Read the model definition and answer for the solid it produces. Units are mm, in the model's axes. A direction names the side the tool comes from. Coordinates: 2 decimals unless noted, no trailing zeros. Order: outer loops, then holes, each group sorted by start corner. A loop starts at its lowest first (then second) coordinate and runs counter-clockwise, first axis right, second up. Notation, with made-up numbers: (-24.5, 31) -> (30.5, 31) arc R26 cw to (30.5, 56) -> close; hole circle Ø4 at (50, -8). An arc over 180 degrees is marked (long way). Answer in a Markdown table with one row per item.
Autodesk Inventor part; units mm, degrees
ref_plane "YZ Plane" through (0, 0, 0) normal (1, 0, 0) x (0, 1, 0)
ref_plane "XZ Plane" through (0, 0, 0) normal (0, 1, 0) x (-1, 0, 0)
ref_plane "XY Plane" through (0, 0, 0) normal (0, 0, 1) x (1, 0, 0)
sketch "Sketch1" plane through (0, 0, 0) normal (0, 0, 1) x (1, 0, 0)
  line L0 (-50, 0) -> (50, 0)
  line L1 (0, 0) -> (0, 34.9563) construction
  line L2 (-50, 0) -> (-50, 10)
  line L3 (-50, 10) -> (50, 10)
  line L4 (50, 10) -> (50, 0)
  dimension "d0" = 100
  dimension "d1" = 10
revolve "Revolution1" add sketch "Sketch1" angle 360 about axis through (-50, 0, 0) along (1, 0, 0)
sketch "Sketch2" plane through (0, 0, 0) normal (0, 1, 0) x (-1, 0, 0)
  line L0 (-50, 10) -> (-50, -10)
  circle A0 centre (-50, 0) radius 17.5
  circle A1 centre (-50, 0) radius 10
  point P0 (0, 0)
  dimension "d3" = 35
  dimension "d4" = 20
extrude "Extrusion1" add sketch "Sketch2" along normal blind 20
extrude "Extrusion2" cut sketch "Sketch2" against normal blind 20 contours A1 L0 | A0 picked at (-47.9217, -2.6061)
extrude "Extrusion3" cut sketch "Sketch2" along normal blind 20 contours A1 L0 picked at (-47.9217, -2.6061)
sketch "Sketch4" plane through (0, 0, 0) normal (0, 1, 0) x (-1, 0, 0)
  line L0 (50, 10) -> (50, -10)
  circle A0 centre (50, 0) radius 17.5
  circle A1 centre (50, 0) radius 10
  point P0 (0, 0)
  dimension "d17" = 35
  dimension "d18" = 20
extrude "Extrusion6" add sketch "Sketch4" against normal blind 20
extrude "Extrusion7" cut sketch "Sketch4" along normal blind 20 contours L0 A1 | A0 picked at (46.9919, -2.3982)
extrude "Extrusion8" cut sketch "Sketch4" against normal blind 20 contours L0 A1 picked at (46.9919, -2.3982)
Q1. The part is cut by section B-B (z = 0). Write down the section's boundary in (x, y), then the cut area to 3 significant figures.
Outcome:
| item | result |
|---|---|
| outline | (-67.5, -20) -> (-60, -20) -> (-60, 0) -> (-67.5, 0) -> close; (-40, -20) -> (-32.5, -20) -> (-32.5, -10) -> (32.5, -10) -> (32.5, 0) -> (40, 0) -> (40, 20) -> (32.5, 20) -> (32.5, 10) -> (-32.5, 10) -> (-32.5, 0) -> (-40, 0) -> close; (60, 0) -> (67.5, 0) -> (67.5, 20) -> (60, 20) -> close |
| area | 1,900 mm² |
Q2. For faces 1 (the face through (0.5, -2.17, -9.76)), 2 (the face through (32.5, -3.8, -0.1)), 3 (the face through (-32.5, 3.8, -0.1)), determine the directions among +Z, -Z, +X, -X, +Y, -Y from which every point of the face is accessible in a straight line to the end or side of a thin tool.
Outcome:
| item | result |
|---|---|
| face 1 | none |
| face 2 | +X, -Y |
| face 3 | -X, +Y |
Q3. Consider line 1 (Z direction, x = 50, y = 6); line 2 (X direction, y = -7.75, z = 0); line 3 (X direction, y = 15, z = 0). Determine where each line is inside the solid, lowest interval first.
Outcome:
| item | result |
|---|---|
| line 1 | -17.5 to -10, 10 to 17.5 |
| line 2 | -67.5 to -60, -40 to 32.5 |
| line 3 | 32.5 to 40, 60 to 67.5 |
Q4. Given pin 1 (17.5 mm diameter, centred on x = 46, z = 3.5, fed in from -Y); pin 2 (2 mm diameter, centred on x = 28.5, z = 5, fed in from +Y); pin 3 (10 mm diameter, centred on x = -8, z = -8, fed in from -Y), each flat-ended and moving along its own axis, determine where each tip first touches the part or whether it passes through.
Outcome:
| item | result |
|---|---|
| pin 1 | y = 0 |
| pin 2 | y = 9.17 |
| pin 3 | y = -9.54 |
Q5. For a pull along Z with two mould halves and no side action, classify faces 4 (the face through (60, 10, 0)), 5 (the face through (67.483, 9.86, -0.769)), 6 (the face through (42, 20, -8)) as pulls with the +Z half, pulls with the -Z half, needs draft (parallel to the pull), parting line crosses it, or undercut.
Outcome:
| item | result |
|---|---|
| face 4 | undercut |
| face 5 | parting line crosses it |
| face 6 | needs draft |
Q6. The part is cut by section A-A (x = 50). Write down the section's boundary in (y, z).
Outcome:
| item | result |
|---|---|
| outline | (0, -17.5) -> (20, -17.5) -> (20, -10) -> (0, -10) -> close; (0, 10) -> (20, 10) -> (20, 17.5) -> (0, 17.5) -> close |
Q7. The part is cut by section C-C (z = -14). Write down the section's boundary in (x, y).
Outcome:
| item | result |
|---|---|
| outline | (-60.5, -20) -> (-39.5, -20) -> (-39.5, 0) -> (-60.5, 0) -> close; (39.5, 0) -> (60.5, 0) -> (60.5, 20) -> (39.5, 20) -> close |
Q8. The part is cut by section D-D (y = 2). Write down the section's boundary in (x, z), then the cut area to 3 significant figures.
Outcome:
| item | result |
|---|---|
| outline | (-35.5, -9.8) -> (35.5, -9.8) arc R17.5 ccw (long way) to (35.5, 9.8) -> (-35.5, 9.8) arc R17.5 cw to start; hole circle Ø20 at (50, 0) |
| area | 1,960 mm² |
